```python
from build123d import *

# Parameters (mm, degrees)
F0_W     = 181
F0_H     = 167
F1_DEPTH = 76
F2_W     = 45
F2_H     = 20
F3_DEPTH = 20
F4_W     = 45
F4_H     = 20
F5_DEPTH = 20


with BuildPart() as f1:
    # F0 (on Right) → F1 (new body)
    with BuildSketch(Plane.YZ):
        with Locations((-1.121614, 20.87992)):
            Rectangle(F0_W, F0_H)
    extrude(amount=F1_DEPTH)

    # F2 (on face) → F3 (cut)
    with BuildSketch(Plane.YZ.offset(76)):
        with Locations((-69.121614, 94.37992)):
            Rectangle(F2_W, F2_H)
    extrude(amount=-F3_DEPTH, mode=Mode.SUBTRACT)

    # F4 (on face) → F5 (cut)
    with BuildSketch(Plane.YZ.offset(76)):
        with Locations((66.878386, 94.37992)):
            Rectangle(F4_W, F4_H)
    extrude(amount=-F5_DEPTH, mode=Mode.SUBTRACT)


solid = f1.part
```
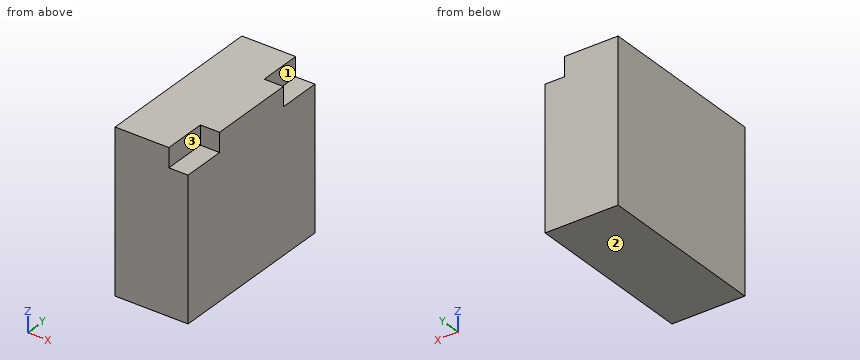
Geometry: final body of the model. Coordinates: model frame, mm. Face numbers are marked on the shaded views. A direction names the side the tool comes from. Coordinates: 2 decimals unless noted, no trailing zeros. Order: outer loops, then holes, each group sorted by start corner. A loop starts at its lowest first (then second) coordinate and runs counter-clockwise, first axis right, second up. Notation, with made-up numbers: M -8.75,-15.75 L 24.25,-15.75 A36 ccw 24.25,23.25 Z; hole C 65,13.25 d5. An arc over 180 degrees is marked long. Answer as CSV lines item,"result".
Q1. Section A-A on x = 64. Return the cut outline in (y, z).
Answers:
outline,"M -91.62,-62.62 L 89.38,-62.62 L 89.38,84.38 L 44.38,84.38 L 44.38,104.38 L -46.62,104.38 L -46.62,84.38 L -91.62,84.38 Z"
Q2. First-contact query: P1, Ø6, axis at y = 71, z = 99, coming from the +X side; P2, Ø16, axis at x = 68, y = 69.5, coming from the +Z side. Flat tips, straight axial feed; report the tip coordinate or a pass-through.
Answers:
P1,"stops at x = 56"
P2,"stops at z = 84.38"
Q3. Section B-B on y = -73.5. Return the cut outline in (x, z), and give its area (3 significant figures).
Answers:
outline,"M 0,-62.62 L 76,-62.62 L 76,84.38 L 56,84.38 L 56,104.38 L 0,104.38 Z"
area,"12,300 mm^2"
Q4. Line query: probe 1 along Z at (x, y) = (70, -82). Output: solid intervals per line, ascending. Write a range as [from, to].
Answers:
probe 1,"z = [-62.62, 84.38]"
Q5. Set-up query: the marked faces 1, 2 and 3. Return all of +Z, -Z, +X, -X, +Y, -Y with unobstructed straight access to the full face (end or side cutting, diameter ignored); none if empty.
Answers:
face 1,"+Z, +X, +Y"
face 2,"-Z, +X, -X, +Y, -Y"
face 3,"+Z, +X, -Y"
